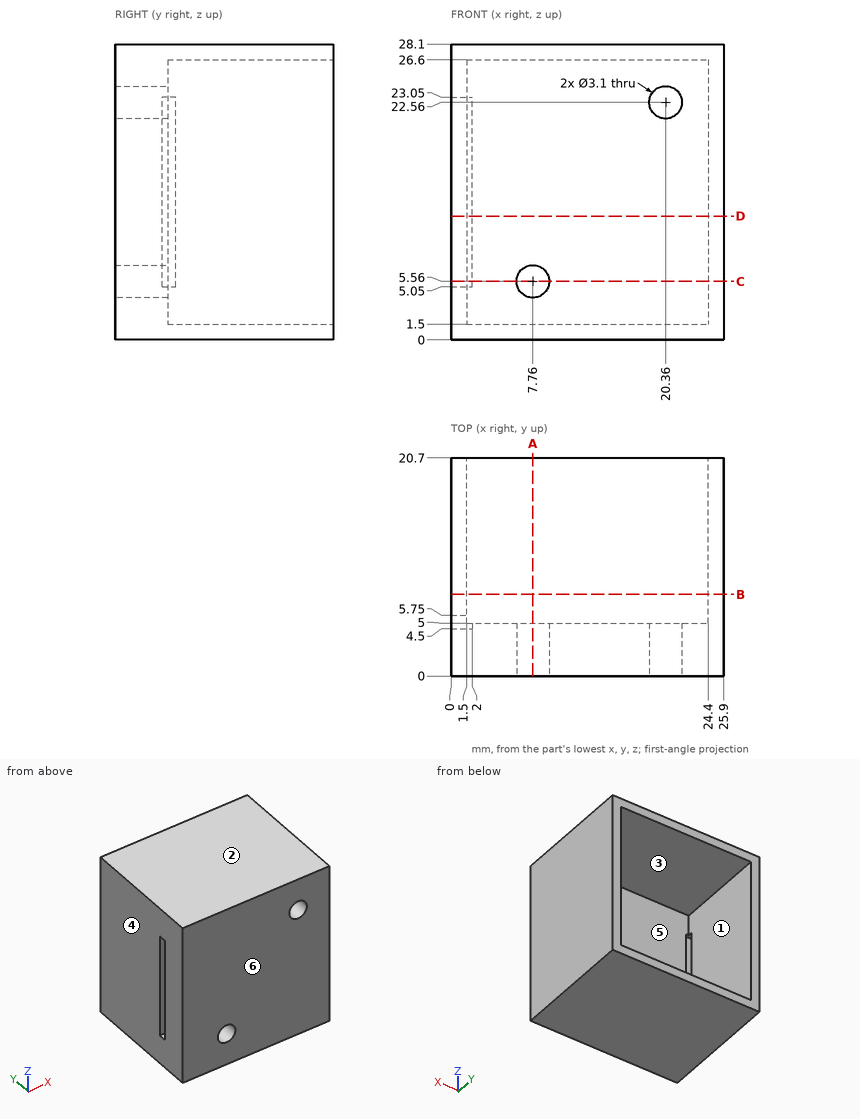
Geometry check sheet. Reference: drawing and pictorial views, mm from the part's lowest x, y, z. A direction names the side the tool comes from. Coordinates: 2 decimals unless noted, no trailing zeros. Loops run counter-clockwise (first coordinate to the right, second up) from the corner with the lowest first, then second, coordinate; pieces in that order, holes last. Notation, with made-up numbers: (34, 44.25) -> (85, 44.25) arc R18 cw to (85, 51.25) -> close; hole circle Ø8 at (74.5, 40). An arc over 180 degrees is marked (long way). Put each result on its own line as item: value.
1) Cross-section at C-C on z = 5.56. Record the boundary of the cut face in (x, y).
Result set:
outline: (0, 0) -> (6.21, 0) -> (6.21, 5) -> (2, 5) -> (2, 4.5) -> (0, 4.5) -> close; (0, 5.75) -> (1.5, 5.75) -> (1.5, 20.7) -> (0, 20.7) -> close; (9.31, 0) -> (25.9, 0) -> (25.9, 20.7) -> (24.4, 20.7) -> (24.4, 5) -> (9.31, 5) -> close
2) Release check for a two-part mould opening along Z. For the marked faces 1, 2, 3 and 4 record: released by +Z, released by -Z, zero draft, split by the parting line, or undercut.
Result set:
face 1: undercut
face 2: released by +Z
face 3: undercut
face 4: zero draft
3) Thickness scan on line 1 (X direction, y = 15.5, z = 11.5); line 2 (X direction, y = 3.2, z = 5.56); line 3 (Z direction, x = 5.25, y = 7.25). Record the ranges inside material, lowest first.
Result set:
line 1: x = 0 to 1.5, 24.4 to 25.9
line 2: x = 0 to 6.21, 9.31 to 25.9
line 3: z = 0 to 1.5, 26.6 to 28.1
4) Tool access check on the marked faces 5 and 6. Record the directions out of +Z, -Z, +X, -X, +Y, -Y that give a thin tool (end or side, any length) a straight path to the whole face; none if there is none.
Result set:
face 5: +Y
face 6: +Z, -Z, +X, -X, -Y
5) Cross-section at D-D on z = 11.75. Record the boundary of the cut face in (x, y).
Result set:
outline: (0, 0) -> (25.9, 0) -> (25.9, 20.7) -> (24.4, 20.7) -> (24.4, 5) -> (2, 5) -> (2, 4.5) -> (0, 4.5) -> close; (0, 5.75) -> (1.5, 5.75) -> (1.5, 20.7) -> (0, 20.7) -> close
6) Cross-section at A-A on x = 7.76. Record the boundary of the cut face in (y, z), plus the area to 3 significant figures.
Result set:
outline: (0, 0) -> (20.7, 0) -> (20.7, 1.5) -> (5, 1.5) -> (5, 4.01) -> (0, 4.01) -> close; (0, 7.11) -> (5, 7.11) -> (5, 26.6) -> (20.7, 26.6) -> (20.7, 28.1) -> (0, 28.1) -> close
area: 172 mm^2
7) Cross-section at B-B on y = 7.75. Record the boundary of the cut face in (x, z), plus the area to 3 significant figures.
Result set:
outline: (0, 0) -> (25.9, 0) -> (25.9, 28.1) -> (0, 28.1) -> close; hole (1.5, 1.5) -> (24.4, 1.5) -> (24.4, 26.6) -> (1.5, 26.6) -> close
area: 153 mm^2
8) Gauge pin test, flat end, axial feed: pin 1 Ø8 at (x, z) = (12, 21) entering from +Y. Record the tip position at first contact, or that the pin passes through.
Result set:
pin 1: stops at y = 5
